The listing builds one solid part. Answer for the finished solid, in the listing's coordinates (mm). Coordinates: 2 decimals unless noted, no trailing zeros. Loops run counter-clockwise (first coordinate to the right, second up) from the corner with the lowest first, then second, coordinate; pieces in that order, holes last. Notation, with made-up numbers: M 9.25,12 L 22.25,12 A31 cw 22.25,38 Z; hole C -9,7 d8. An arc over 180 degrees is marked long. Answer as a JSON object with one key per item and string values. Group by question number.
1. Straight lines are drawn through the part: L1, parallel to X at y = -119, z = 0; L2, parallel to X at y = 119, z = 8.5. For each, find the intervals that lie inside material, in ascending order.
2. A cutting plane is placed at B-B on z = 0. Give the vertices of the cut face in (x, y).
3. A cutting plane is placed at A-A on y = -164. Give the vertices of the cut face in (x, z), and give its area (3 significant figures).
4. Given pin 1 (2 mm diameter, centred on y = -122, z = 1, fed in from -X); pin 2 (0.6 mm diameter, centred on x = -9, y = -43, fed in from +Z); pin 3 (0.6 mm diameter, centred on y = -121.5, z = -9.5, fed in from -X), each flat-ended and moving along its own axis, determine where each tip first touches the part or whether it passes through.
5. A cutting plane is placed at C-C on x = 0. Give the vertices of the cut face in (y, z), and give its area (3 significant figures).
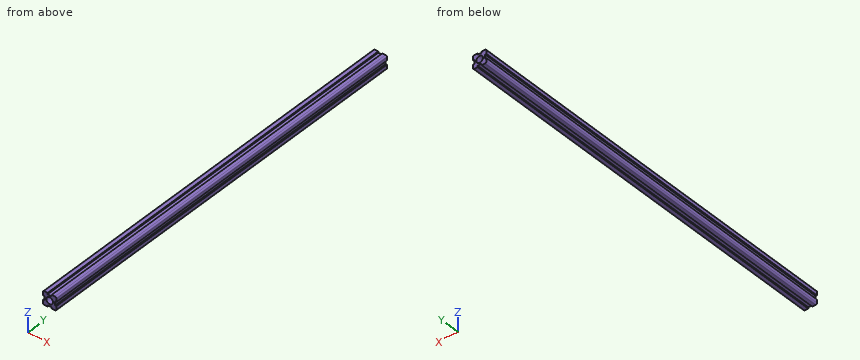
from build123d import *

# Parameters (mm, degrees)
SKETCH1_W           = 20
SKETCH1_H           = 20
SKETCH1_R           = 5
BOSS_EXTRUDE2_DEPTH = 300
SKETCH2_W           = 6
SKETCH2_H           = 4
SKETCH2_W_2         = 4
SKETCH2_H_2         = 6
CUT_EXTRUDE1_DEPTH  = 600
FILLET1_R           = 2


with BuildPart() as part:
    # Sketch1 → Boss-Extrude2 (new body, symmetric)
    with BuildSketch(Plane(origin=(0, 0, 0), x_dir=(1, 0, 0), z_dir=(0, 1, 0))):
        Rectangle(SKETCH1_W, SKETCH1_H)
        Circle(SKETCH1_R, mode=Mode.SUBTRACT)
    extrude(amount=BOSS_EXTRUDE2_DEPTH, both=True)

    # Sketch2 → Cut-Extrude1 (cut)
    with BuildSketch(Plane.XZ.offset(300)):
        with Locations((0, 10)):
            Rectangle(SKETCH2_W, SKETCH2_H)
        with Locations((10, 0)):
            Rectangle(SKETCH2_W_2, SKETCH2_H_2)
        with Locations((0, -10)):
            Rectangle(SKETCH2_W, SKETCH2_H)
        with Locations((-10, 0)):
            Rectangle(SKETCH2_W_2, SKETCH2_H_2)
    extrude(amount=-CUT_EXTRUDE1_DEPTH, mode=Mode.SUBTRACT)

    # Fillet1
    fillet1_edges = [part.edges().sort_by_distance(p)[0] for p in [
        (10, 0, 10),
        (-10, 0, 10),
        (-10, 0, -10),
        (10, 0, -10),
    ]]
    fillet(fillet1_edges, radius=FILLET1_R)


solid = part.part
From the geometry:
{
 "1": {"L1": "x = -8 to -5, 5 to 8", "L2": "x = -9.94 to -3, 3 to 9.94"},
 "2": {"outline": "M -8,-300 L -5,-300 L -5,300 L -8,300 Z; M 5,-300 L 8,-300 L 8,300 L 5,300 Z"},
 "3": {"outline": "M -10,-8 A2 ccw -8,-10 L -3,-10 L -3,-8 L 3,-8 L 3,-10 L 8,-10 A2 ccw 10,-8 L 10,-3 L 8,-3 L 8,3 L 10,3 L 10,8 A2 ccw 8,10 L 3,10 L 3,8 L -3,8 L -3,10 L -8,10 A2 ccw -10,8 L -10,3 L -8,3 L -8,-3 L -10,-3 Z; hole C 0,0 d10", "area": "270 mm²"},
 "4": {"pin 1": "stops at x = -8", "pin 2": "stops at z = 9.87", "pin 3": "stops at x = -9.6"},
 "5": {"outline": "M -300,-8 L 300,-8 L 300,-5 L -300,-5 Z; M -300,5 L 300,5 L 300,8 L -300,8 Z", "area": "3,600 mm²"}
}
